Answer from the drawing. Dimensions are ordinates in mm from the lowest x, y and z of the part. A direction names the side the tool comes from. Round coordinates to 2 decimals unless told otherwise and drop trailing zeros. Loops run counter-clockwise (first coordinate to the right, second up) from the corner with the lowest first, then second, coordinate; pieces in that order, holes last. Notation, with made-up numbers: (70.5, -14) - (82.5, -14) arc R33 ccw to (82.5, 21) - close; hole circle Ø1 at (46, -4.75). An arc over 180 degrees is marked (long way). Answer as CSV lines item,"result". Start each with the question number.
Q1. For the marked faces 1, 2 and 3, determine the directions among +Z, -Z, +X, -X, +Y, -Y from which every point of the face is accessible in a straight line to the end or side of a thin tool.
Q2. Section B-B on x = 55.5 is taken. Write down the section's boundary in (y, z) (1 decimal), then the cut area to 3 significant figures.
Q3. The mould has two halves that part along Y. Classify the marked faces 4, 5, 6 and 7: +Y half, -Y half, draft (parallel to the pull), parting line (faces both ways), or undercut.
Q4. Straight lines are drawn through the part: L1, parallel to Y at x = 60, z = 58; L2, parallel to Y at x = 50, z = 8.5 (1 decimal); L3, parallel to Y at x = 13, z = 57. For each, find the intervals that lie inside material, in ascending order. Write a range as [from, to].
Q5. Section C-C on z = 46.5 is taken. Count the separate pieces of the cut face and the enclosed holes in it, then the cut area to 3 significant figures.
Q6. Section D-D on x = 72 is taken. Write down the section's boundary in (y, z) (1 decimal), then the cut area to 4 significant figures.
Q7. Each of these flat-tipped pins is pushed along its axis until it touches: pin 1 Ø10 at (x, y) = (52.5, 100.5) entering from -Z; pin 2 Ø7.5 at (y, z) = (83.5, 53.5) entering from -X; pin 3 Ø11.5 at (x, z) = (28.5, 20) entering from +Y. Where does it stop, or does it pass through?
Q8. Section A-A on z = 21 is taken. Write down the section's boundary in (x, y) (1 decimal).
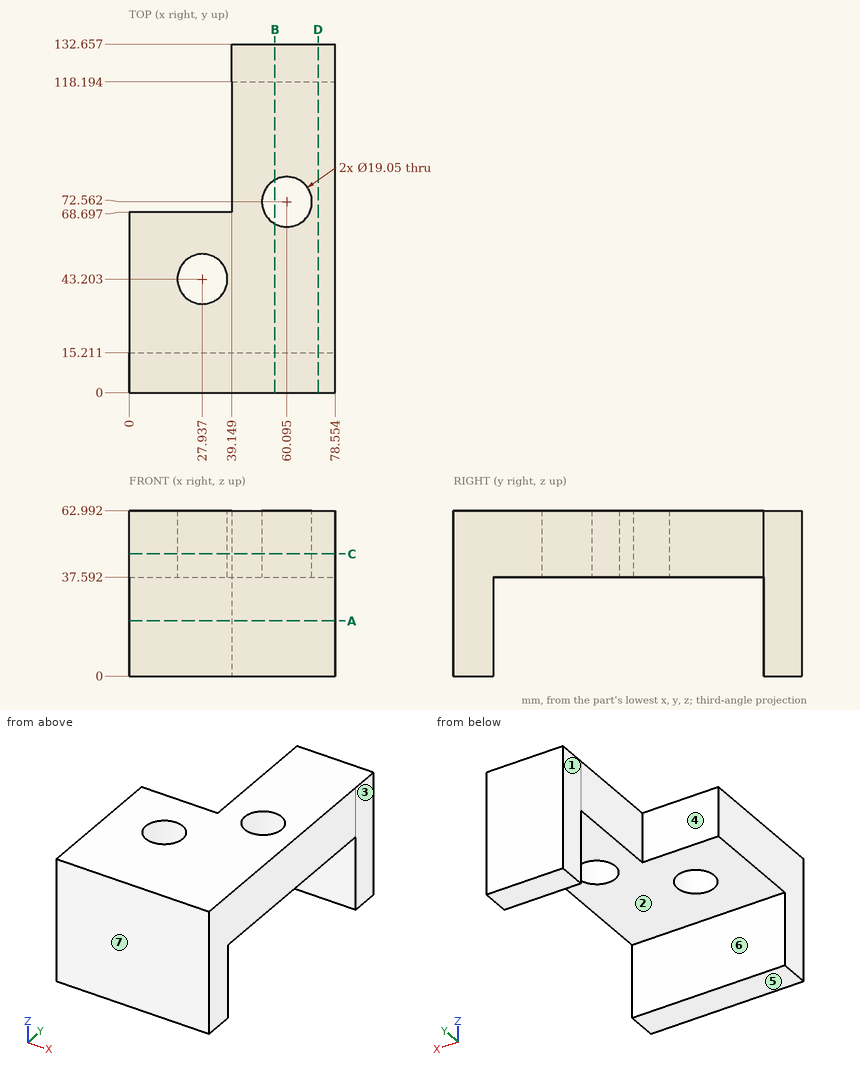
Findings:
1,face 1,"+Z, -Z, -X, +Y"
1,face 2,"-Z, +X, -X"
1,face 3,"+Z, -Z, +X, +Y, -Y"
2,outline,"(0, 0) - (15.2, 0) - (15.2, 37.6) - (64.2, 37.6) - (64.2, 63) - (0, 63) - close; (80.9, 37.6) - (118.2, 37.6) - (118.2, 0) - (132.7, 0) - (132.7, 63) - (80.9, 63) - close"
2,area,"4,060 mm^2"
3,face 4,"+Y half"
3,face 5,"draft"
3,face 6,"undercut"
3,face 7,"-Y half"
4,L1,"y = [0, 63.04], [82.09, 132.66]"
4,L2,"y = [0, 15.2], [118.2, 132.7]"
4,L3,"y = [0, 68.7]"
5,separate pieces,"1"
5,enclosed holes,"2"
5,area,"7,350 mm^2"
6,outline,"(0, 0) - (15.2, 0) - (15.2, 37.6) - (118.2, 37.6) - (118.2, 0) - (132.7, 0) - (132.7, 63) - (0, 63) - close"
6,area,"4,485 mm^2"
7,pin 1,"stops at z = 37.59"
7,pin 2,"stops at x = 39.15"
7,pin 3,"stops at y = 15.21"
8,outline,"(0, 0) - (78.6, 0) - (78.6, 15.2) - (0, 15.2) - close; (39.1, 118.2) - (78.6, 118.2) - (78.6, 132.7) - (39.1, 132.7) - close"
